Here's how the part is built. I have some questions about the finished solid (model axes, mm). A direction names the side the tool comes from. Round coordinates to 2 decimals unless told otherwise and drop trailing zeros. Write each loop counter-clockwise with the first axis right and the second up, starting at its lowest first coordinate (ties: lowest second). Pieces come first, ordered by that corner, then holes. Notation, with made-up numbers: (51, 73.5) - (67, 73.5) arc R21 ccw to (67, 105.5) - close; hole circle Ø1 at (23, -14). An arc over 180 degrees is marked (long way). Write item = value, one per line. Start each with the question number.
Item 1: If we section it at C-C (y = -2.5): Please give me the cut outline in (x, z), and give its area (4 significant figures).
Item 2: If we section it at A-A (z = 10): Please give me the cut outline in (x, y), and give its area (3 significant figures).
Item 3: Which directions (+Z, -Z, +X, -X, +Y, -Y) give clear straight access to the entire face, cutting with the end or side of a thin tool? Please do faces 4 (the face through (-46.07, 46, 25.92)), 5 (the face through (-48.732, 14.048, 5.436)).
Item 4: If I drill on line 1 along Y through (x, z) = (-48.35, 10); line 2 along X through (y, z) = (-19, 18.5); line 3 along Z through (x, y) = (-49.4, 20), over which ranges is the centre line in solid material (lowest first)? Write a range as [from, to].
Item 5: If we section it at B-B (z = 27): Please give me the cut outline in (x, y).
Item 6: Thinking about a two-plate mould opening in Z: for faces 1 (the face through (-4, -48, 50)), 2 (the face through (47.5, -1, 26)), 3 (the face through (-48.73, -31.63, 2.68)), which applies, pulls with the +Z half, pulls with the -Z half, needs draft (parallel to the pull), parting line crosses it, or undercut?
Item 7: For P1, Ø2, axis at x = 23, y = 3.5, coming from the +Z side; P2, Ø1, axis at x = -33.5, y = -32, coming from the -Z side, each with a flat end and sliding along its axis, tell me the tip position at first contact or that it passes through.
```python
from build123d import *

# Parameters (mm, degrees)
F0_W     = 100
F0_H     = 100
F1_DEPTH = 50
F2_T     = -2.5
F3_R     = 5
F4_R     = 7.5
F5_DEPTH = 100.001


with BuildPart() as f1:
    # F0 (on Top) → F1 (new body)
    with BuildSketch(Plane.XY):
        Rectangle(F0_W, F0_H)
    extrude(amount=F1_DEPTH)

    # F2
    f2_openings = [f1.faces().sort_by_distance(p)[0] for p in [
        (0, 0, 50),
    ]]
    offset(amount=F2_T, openings=f2_openings)

    # F3
    f3_edges = [f1.edges().sort_by_distance(p)[0] for p in [
        (-47.5, 47.5, 26.25),
        (47.5, 47.5, 26.25),
        (-47.5, -47.5, 26.25),
        (47.5, -47.5, 26.25),
    ]]
    fillet(f3_edges, radius=F3_R)

    # F4 (on face) → F5 (cut, through all)
    with BuildSketch(Plane.YZ.offset(50)):
        with Locations((-30, 10)):
            Circle(F4_R)
        with Locations((20, 10)):
            Circle(F4_R)
    extrude(amount=-F5_DEPTH, mode=Mode.SUBTRACT)


solid = f1.part
```
Reply:
q1.outline = (-50, 0) - (50, 0) - (50, 50) - (47.5, 50) - (47.5, 2.5) - (-47.5, 2.5) - (-47.5, 50) - (-50, 50) - close
q1.area = 487.5 mm2
q2.outline = (-50, -50) - (50, -50) - (50, -37.5) - (47.5, -37.5) - (47.5, -42.5) arc R5 cw to (42.5, -47.5) - (-42.5, -47.5) arc R5 cw to (-47.5, -42.5) - (-47.5, -37.5) - (-50, -37.5) - close; (-50, -22.5) - (-47.5, -22.5) - (-47.5, 12.5) - (-50, 12.5) - close; (-50, 27.5) - (-47.5, 27.5) - (-47.5, 42.5) arc R5 cw to (-42.5, 47.5) - (42.5, 47.5) arc R5 cw to (47.5, 42.5) - (47.5, 27.5) - (50, 27.5) - (50, 50) - (-50, 50) - close; (47.5, -22.5) - (50, -22.5) - (50, 12.5) - (47.5, 12.5) - close
q2.area = 846 mm2
q3.face_4 = +Z
q3.face_5 = +X, -X
q4.line_1 = [-50, -37.5], [-22.5, 12.5], [27.5, 50]
q4.line_2 = [-50, -47.5], [47.5, 50]
q4.line_3 = [0, 2.5], [17.5, 50]
q5.outline = (-50, -50) - (50, -50) - (50, 50) - (-50, 50) - close; hole (-47.5, -42.5) arc R5 ccw to (-42.5, -47.5) - (42.5, -47.5) arc R5 ccw to (47.5, -42.5) - (47.5, 42.5) arc R5 ccw to (42.5, 47.5) - (-42.5, 47.5) arc R5 ccw to (-47.5, 42.5) - close
q6.face_1 = pulls with the +Z half
q6.face_2 = needs draft
q6.face_3 = undercut
q7.P1 = 2.5
q7.P2 = 0
